Can you work these out from the drawing? Everything is in mm from the part's minimum corner. Coordinates: 2 decimals unless noted, no trailing zeros. Order: outer loops, then holes, each group sorted by start corner. A loop starts at its lowest first (then second) coordinate and runs counter-clockwise, first axis right, second up. Notation, with made-up numbers: M 20,6.25 L 48,6.25 A20 ccw 48,38.25 Z; hole C 31.25,-16 d7. An arc over 180 degrees is marked long. Answer as a JSON object with one key per item and string values.
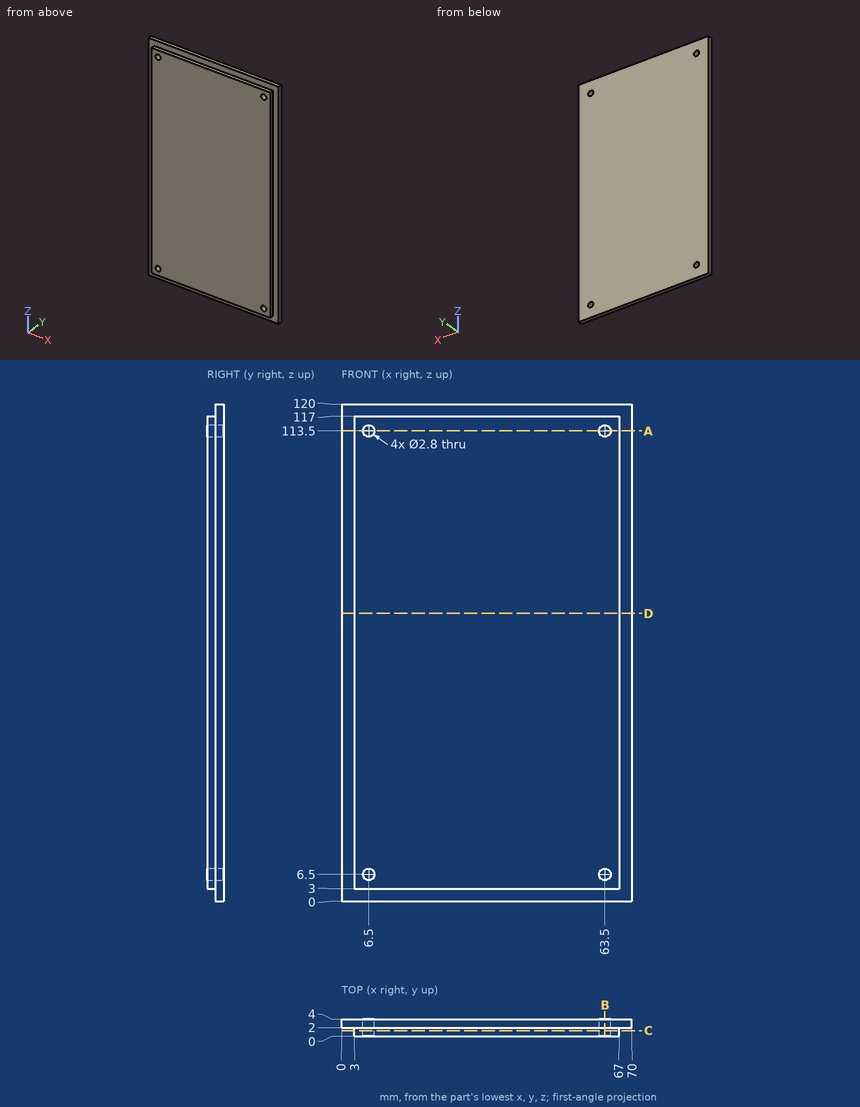
Item 1: I want a section at C-C, the plane y = 1.3. Write out the boundary of the cut face in (x, z), plus the area to 3 significant figures.
Answers follow:
{"outline": "M 3,3 L 67,3 L 67,117 L 3,117 Z; hole C 6.5,6.5 d2.8; hole C 6.5,113.5 d2.8; hole C 63.5,6.5 d2.8; hole C 63.5,113.5 d2.8", "area": "7,270 mm^2"}
Item 2: I want a section at B-B, the plane x = 63.5. Write out the boundary of the cut face in (y, z), plus the area to 3 significant figures.
Answers follow:
{"outline": "M 0,3 L 2,3 L 2,0 L 4,0 L 4,5.1 L 0,5.1 Z; M 0,7.9 L 4,7.9 L 4,112.1 L 0,112.1 Z; M 0,114.9 L 4,114.9 L 4,120 L 2,120 L 2,117 L 0,117 Z", "area": "446 mm^2"}
Item 3: I want a section at A-A, the plane z = 113.5. Write out the boundary of the cut face in (x, y).
Answers follow:
{"outline": "M 0,2 L 3,2 L 3,0 L 5.1,0 L 5.1,4 L 0,4 Z; M 7.9,0 L 62.1,0 L 62.1,4 L 7.9,4 Z; M 64.9,0 L 67,0 L 67,2 L 70,2 L 70,4 L 64.9,4 Z"}
Item 4: I'm going to push flat-ended pins straight in: pin 1 (1.5 mm diameter, centred on x = 59, y = 3.5, fed in from -Z); pin 2 (2.5 mm diameter, centred on x = 6.5, z = 6.5, fed in from -Y); pin 3 (2 mm diameter, centred on x = 37, y = 0.5, fed in from -Z). Where does each tip first touch, or does it pass through?
Answers follow:
{"pin 1": "stops at z = 0", "pin 2": "passes through", "pin 3": "stops at z = 3"}
Item 5: Please list where these lines run through material, in increasing order: line 1 (X direction, y = 2.95, z = 113.5); line 2 (X direction, y = 1.4, z = 6.5); line 3 (X direction, y = 0.5, z = 54.5).
Answers follow:
{"line 1": "x = 0 to 5.1, 7.9 to 62.1, 64.9 to 70", "line 2": "x = 3 to 5.1, 7.9 to 62.1, 64.9 to 67", "line 3": "x = 3 to 67"}
Item 6: I want a section at D-D, the plane z = 69.5. Write out the boundary of the cut face in (x, y), plus the area to 3 significant figures.
Answers follow:
{"outline": "M 0,2 L 3,2 L 3,0 L 67,0 L 67,2 L 70,2 L 70,4 L 0,4 Z", "area": "268 mm^2"}
